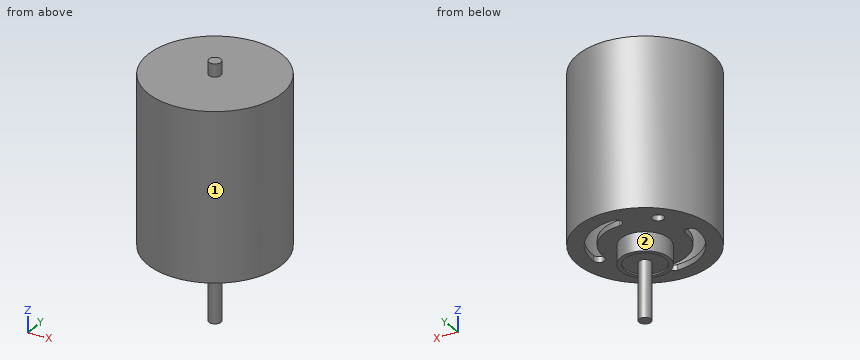
```python
from build123d import *

# Parameters (mm, degrees)
SKETCH3_W          = 1.5875
SKETCH3_H          = 68.218126879
SKETCH4_W          = 16.5
SKETCH4_H          = 42
CUT_EXTRUDE1_REACH = 56.738
SKETCH5_R          = 1.5


with BuildPart() as part:
    # Sketch2 → Revolve1 (revolve)
    with BuildSketch(Plane(origin=(0, 0, 0), x_dir=(1, 0, 0), z_dir=(0, 1, 0)), mode=Mode.PRIVATE) as revolve1_sk:
        Polygon((0, 0), (18, 0), (18, 45), (6.5, 45), (6.5, 50), (5.455078682, 50), (5.455078682, 49.6), (0, 49.6), align=None)
    revolve(revolve1_sk.sketch.rotate(Axis((0, 0, -54.973870739), (0, 0, 1)), 180), axis=Axis((0, 0, -54.973870739), (0, 0, 1)))

    # Sketch3 → Revolve-Thin1 (revolve)
    with BuildSketch(Plane(origin=(0, 0, 0), x_dir=(1, 0, 0), z_dir=(0, 1, 0)), mode=Mode.PRIVATE) as revolve_thin1_sk:
        with Locations((-0.79375, 30.65040302)):
            Rectangle(SKETCH3_W, SKETCH3_H)
    revolve(revolve_thin1_sk.sketch.rotate(Axis((0, 0, 0), (0, 0, -1)), 180), axis=Axis((0, 0, 0), (0, 0, -1)))

    # Sketch4 → Cut-Revolve2 (revolve, cut)
    with BuildSketch(Plane(origin=(0, 0, 0), x_dir=(1, 0, 0), z_dir=(0, 1, 0))):
        with Locations((8.25, 22.5)):
            Rectangle(SKETCH4_W, SKETCH4_H)
    revolve(axis=Axis((0, 0, 0), (0, 0, -1)), mode=Mode.SUBTRACT)

    # Sketch5 → Cut-Extrude1 (cut, up to next)
    with BuildSketch(Plane(origin=(0, 0, -45), x_dir=(-1, 0, 0), z_dir=(0, 0, -1)), mode=Mode.PRIVATE) as cut_extrude1_sk1:
        with Locations((9.545941546, 9.545941546)):
            Circle(SKETCH5_R)
    cut_extrude1_tool1 = extrude(cut_extrude1_sk1.sketch, amount=-CUT_EXTRUDE1_REACH, mode=Mode.PRIVATE) & part.part
    # Sketch5 → Cut-Extrude1 (cut, up to next)
    with BuildSketch(Plane(origin=(0, 0, -45), x_dir=(-1, 0, 0), z_dir=(0, 0, -1)), mode=Mode.PRIVATE) as cut_extrude1_sk2:
        with Locations((-9.545941546, -9.545941546)):
            Circle(SKETCH5_R)
    cut_extrude1_tool2 = extrude(cut_extrude1_sk2.sketch, amount=-CUT_EXTRUDE1_REACH, mode=Mode.PRIVATE) & part.part
    # Sketch5 → Cut-Extrude1 (cut, up to next)
    with BuildSketch(Plane(origin=(0, 0, -45), x_dir=(-1, 0, 0), z_dir=(0, 0, -1)), mode=Mode.PRIVATE) as cut_extrude1_sk3:
        with BuildLine():
            ThreePointArc((0, 14), (-9.899494937, 9.899494937), (-14, 0))
            ThreePointArc((-14, 0), (-12.5, -1.5), (-11, 0))
            ThreePointArc((-11, 0), (-7.778174593, 7.778174593), (0, 11))
            ThreePointArc((0, 11), (1.5, 12.5), (0, 14))
        make_face()
    cut_extrude1_tool3 = extrude(cut_extrude1_sk3.sketch, amount=-CUT_EXTRUDE1_REACH, mode=Mode.PRIVATE) & part.part
    # Sketch5 → Cut-Extrude1 (cut, up to next)
    with BuildSketch(Plane(origin=(0, 0, -45), x_dir=(-1, 0, 0), z_dir=(0, 0, -1)), mode=Mode.PRIVATE) as cut_extrude1_sk4:
        with BuildLine():
            ThreePointArc((14, 0), (9.899494937, -9.899494937), (0, -14))
            ThreePointArc((0, -14), (-1.5, -12.5), (0, -11))
            ThreePointArc((0, -11), (7.778174593, -7.778174593), (11, 0))
            ThreePointArc((11, 0), (12.5, 1.5), (14, 0))
        make_face()
    cut_extrude1_tool4 = extrude(cut_extrude1_sk4.sketch, amount=-CUT_EXTRUDE1_REACH, mode=Mode.PRIVATE) & part.part
    add(cut_extrude1_tool1.solids().sort_by_distance((-9.545942, 9.545942, -45))[0], mode=Mode.SUBTRACT)
    add(cut_extrude1_tool2.solids().sort_by_distance((9.545942, -9.545942, -45))[0], mode=Mode.SUBTRACT)
    add(cut_extrude1_tool3.solids().sort_by_distance((12.5, -1.280797, -45))[0], mode=Mode.SUBTRACT)
    add(cut_extrude1_tool4.solids().sort_by_distance((-7.933175, -7.933175, -45))[0], mode=Mode.SUBTRACT)


solid = part.part
```
For this review, take the finished solid that the model builds, in its own axes (mm). Face numbers are marked on the shaded views. A direction names the side the tool comes from. Coordinates: 2 decimals unless noted, no trailing zeros. Order: outer loops, then holes, each group sorted by start corner. A loop starts at its lowest first (then second) coordinate and runs counter-clockwise, first axis right, second up. Notation, with made-up numbers: (53, 89) - (77, 89) arc R12 cw to (77, 101) - close; hole circle Ø1 at (47.5, 50.25). An arc over 180 degrees is marked (long way). Answer as a JSON object with one key per item and string values. Group by question number.
1. We need section A-A on x = 15.5. State the section outline as (y, z) points, then the cut area to 3 significant figures.
2. We need section D-D on z = -17.5. State the section outline as (x, y) points.
3. We need section C-C on y = 4. State the section outline as (x, z) points.
4. For probe 1 along X at (y, z) = (-0.5, -21); probe 2 along Z at (x, y) = (5, 7); probe 3 along Z at (x, y) = (-2, -5), list the stretches that pass through material, from the lowest coordinate up.
5. We need section B-B on x = -12.5. State the section outline as (y, z) points, then the cut area to 3 significant figures.
6. Clearance check with flat-ended pins moving along their axes: P1, Ø6, axis at x = -11, y = 12, coming from the -Z side; P2, Ø4, axis at y = 13.5, z = -35, coming from the -X side; P3, Ø3.5, axis at x = -9.55, y = 9.55, coming from the +Z side. State where each tip first meets the part, or that it passes through.
7. For the marked faces 1 and 2, list the 3-axis set-ups (+Z, -Z, +X, -X, +Y, -Y) from which the entire face can be reached by the end or side of a thin tool; tool diameter is ignored.
Final values:
{
 "1": {"outline": "(-9.15, -45) - (9.15, -45) - (9.15, 0) - (-9.15, 0) - close; hole (-5.66, -43.5) - (5.66, -43.5) - (5.66, -1.5) - (-5.66, -1.5) - close", "area": "348 mm²"},
 "2": {"outline": "circle Ø36 at (0, 0); hole circle Ø33 at (0, 0)"},
 "3": {"outline": "(-17.55, -45) - (-5.12, -45) - (-5.12, -50) - (-3.71, -50) - (-3.71, -49.6) - (3.71, -49.6) - (3.71, -50) - (5.12, -50) - (5.12, -45) - (10.25, -45) - (10.25, -43.5) - (-16.01, -43.5) - (-16.01, -1.5) - (16.01, -1.5) - (16.01, -43.5) - (13.42, -43.5) - (13.42, -45) - (17.55, -45) - (17.55, 0) - (-17.55, 0) - close"},
 "4": {"probe 1": "-17.99 to -16.49, 16.49 to 17.99", "probe 2": "-45 to -43.5, -1.5 to 0", "probe 3": "-49.6 to -43.5, -1.5 to 0"},
 "5": {"outline": "(-12.95, -45) - (-6.3, -45) - (-6.3, -43.5) - (-10.77, -43.5) - (-10.77, -1.5) - (10.77, -1.5) - (10.77, -43.5) - (1.5, -43.5) - (1.5, -45) - (12.95, -45) - (12.95, 0) - (-12.95, 0) - close", "area": "249 mm²"},
 "6": {"P1": "z = -45", "P2": "x = -13.85", "P3": "z = 0"},
 "7": {"face 1": "+Z, -Z", "face 2": "-Z"}
}
